Check sheet for the modelled part. Datum: model origin and axes. Units: mm. Face numbers are marked on the shaded views. A direction names the side the tool comes from. Give positions to 0.01 mm unless a question says otherwise; leave off trailing zeros. Loops run counter-clockwise (first coordinate to the right, second up) from the corner with the lowest first, then second, coordinate; pieces in that order, holes last. Notation, with made-up numbers: (39, -2.5) -> (85, -2.5) arc R22 ccw to (85, 20.5) -> close; hole circle Ø7 at (67, 59). An arc over 180 degrees is marked (long way). Write each question's results on one line, items separated by ' | '. Start each with the question number.
1. Mould release check, pull along Y, two halves, no side actions. Record for the marked faces 4, 5 and 6: +Y half, -Y half, draft (parallel to the pull), parting line (faces both ways), or undercut.
2. Cross-section at A-A on z = 0. Record the boundary of the cut face in (x, y), and give its area (3 significant figures).
3. Cross-section at C-C on z = 9. Record the boundary of the cut face in (x, y), and give its area (3 significant figures).
4. Tool access check on the marked faces 1, 2 and 3. Record the directions out of +Z, -Z, +X, -X, +Y, -Y that give a thin tool (end or side, any length) a straight path to the whole face; none if there is none.
5. Gauge pin test, flat ends, axial feed: pin 1 Ø1 at (x, z) = (1, -3.5) entering from -Y; pin 2 Ø6.5 at (y, z) = (0, 0) entering from -X; pin 3 Ø2 at (x, y) = (3, -9) entering from +Z; pin 4 Ø1.2 at (x, z) = (3, -0.5) entering from -Y. Record the tip position at first contact, or that the pin passes through.
6. Cross-section at B-B on y = 0. Record the boundary of the cut face in (x, z), and give its area (3 significant figures).
7. Cross-section at D-D on y = -3.5. Record the boundary of the cut face in (x, z).
8. Material ranges on L1, parallel to Z at x = 1.25, y = 0; L2, parallel to Y at x = 0.7, z = -0.5; L3, parallel to Y at x = 0.8, z = -7.5, recorded low to high. Write a range as from..to.
Autodesk Inventor part; units mm, degrees
ref_plane "YZ Plane" through (0, 0, 0) normal (1, 0, 0) x (0, 1, 0)
ref_plane "XZ Plane" through (0, 0, 0) normal (0, 1, 0) x (-1, 0, 0)
ref_plane "XY Plane" through (0, 0, 0) normal (0, 0, 1) x (1, 0, 0)
sketch "Эскиз1" plane through (0, 0, 0) normal (1, 0, 0) x (0, 1, 0)
  circle A0 centre (0, 0) radius 12.5
  line L0 (12.339, 2) -> (7.339, 2)
  line L1 (7.339, 2) -> (7.339, -2)
  line L2 (7.339, -2) -> (12.339, -2)
  line L3 (12.5, 0) -> (0, 0)
  line L4 (4.4374, 11.6859) -> (1.9374, 7.3557)
  line L5 (1.9374, 7.3557) -> (5.4015, 5.3557)
  line L6 (5.4015, 5.3557) -> (7.9015, 9.6859)
  line L7 (-7.9015, 9.6859) -> (-5.4015, 5.3557)
  line L8 (-5.4015, 5.3557) -> (-1.9374, 7.3557)
  line L9 (-1.9374, 7.3557) -> (-4.4374, 11.6859)
  line L10 (-12.339, -2) -> (-7.339, -2)
  line L11 (-7.339, -2) -> (-7.339, 2)
  line L12 (-7.339, 2) -> (-12.339, 2)
  line L13 (-4.4374, -11.6859) -> (-1.9374, -7.3557)
  line L14 (-1.9374, -7.3557) -> (-5.4015, -5.3557)
  line L15 (-5.4015, -5.3557) -> (-7.9015, -9.6859)
  line L16 (7.9015, -9.6859) -> (5.4015, -5.3557)
  line L17 (5.4015, -5.3557) -> (1.9374, -7.3557)
  line L18 (1.9374, -7.3557) -> (4.4374, -11.6859)
  circle A1 centre (0, 0) radius 2
  point P0 (4.4374, 11.6859)
  point P1 (-12.339, 2)
  point P2 (-12.339, -2)
  point P3 (-7.9015, -9.6859)
  point P4 (-4.4374, -11.6859)
  point P5 (4.4374, -11.6859)
  point P6 (7.9015, 9.6859)
  dimension "d2" = 360
  dimension "d4" = 5
  dimension "d5" = 25
  dimension "d8" = 4
  dimension "d9" = 4
extrude "Выдавливание1" add sketch "Эскиз1" along normal blind 4 contours L0 L1 L2 A0 L16 L17 L18 L13 L14 L15 L10 L11 L12 L7 L8 L9 L4 L5 L6
properties part number "barrel_holder"
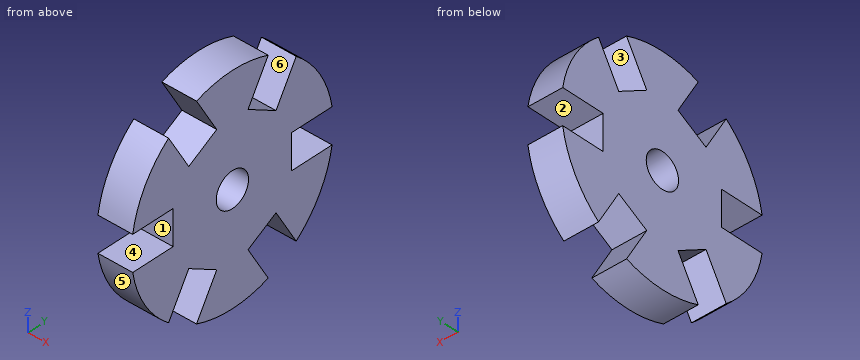
Geometry says:
1) face 4: draft | face 5: -Y half | face 6: undercut
2) outline: (0, -7.34) -> (4, -7.34) -> (4, -2) -> (0, -2) -> close; (0, 2) -> (4, 2) -> (4, 7.34) -> (0, 7.34) -> close | area: 42.7 mm^2
3) outline: (0, -8.67) -> (4, -8.67) -> (4, -7.51) -> (0, -7.51) -> close; (0, -2.89) -> (4, -2.89) -> (4, 2.89) -> (0, 2.89) -> close; (0, 7.51) -> (4, 7.51) -> (4, 8.67) -> (0, 8.67) -> close | area: 32.4 mm^2
4) face 1: +X, -X, -Y | face 2: +X, -X, +Y | face 3: +X, -X
5) pin 1: y = -12.13 | pin 2: x = 0 | pin 3: z = 9.6 | pin 4: y = -7.34
6) outline: (0, -12.5) -> (4, -12.5) -> (4, -2) -> (0, -2) -> close; (0, 2) -> (4, 2) -> (4, 12.5) -> (0, 12.5) -> close | area: 84.0 mm^2
7) outline: (0, -12) -> (4, -12) -> (4, -10.06) -> (0, -10.06) -> close; (0, -6.45) -> (4, -6.45) -> (4, 6.45) -> (0, 6.45) -> close; (0, 10.06) -> (4, 10.06) -> (4, 12) -> (0, 12) -> close
8) L1: -12.5..-2, 2..12.5 | L2: -7.34..-1.94, 1.94..7.34 | L3: -10..-6.64, -2.02..2.02, 6.64..10
